```python
from build123d import *

# Parameters (mm, degrees)
SKETCH_W     = 95
SKETCH_H     = 69
SKETCH_R     = 1.5
PAD_DEPTH    = 3
SKETCH001_R  = 4
PAD001_DEPTH = 4
SKETCH002_R  = 1.45
POCKET_DEPTH = 5


with BuildPart() as part:
    # Sketch → Pad (new body)
    with BuildSketch(Plane.XY):
        Rectangle(SKETCH_W, SKETCH_H)
        with Locations((-44, -31)):
            Circle(SKETCH_R, mode=Mode.SUBTRACT)
        with Locations((44, 31)):
            Circle(SKETCH_R, mode=Mode.SUBTRACT)
    extrude(amount=PAD_DEPTH)

    # Sketch001 (on Face8 of Pad) → Pad001 (join)
    with BuildSketch(Plane.XY.offset(3)):
        with Locations((-36.5, 24)):
            Circle(SKETCH001_R)
        with Locations((-36.5, -24)):
            Circle(SKETCH001_R)
        with Locations((36.5, -24)):
            Circle(SKETCH001_R)
        with Locations((36.5, 24)):
            Circle(SKETCH001_R)
    extrude(amount=PAD001_DEPTH)

    # Sketch002 (on Face14 of Pad001) → Pocket (cut)
    with BuildSketch(Plane.XY.offset(7)):
        with Locations((-36.5, 24)):
            Circle(SKETCH002_R)
        with Locations((-36.5, -24)):
            Circle(SKETCH002_R)
        with Locations((36.5, 24)):
            Circle(SKETCH002_R)
        with Locations((36.5, -24)):
            Circle(SKETCH002_R)
    extrude(amount=-POCKET_DEPTH, mode=Mode.SUBTRACT)


solid = part.part
```
For this review, take the finished solid that the model builds, in its own axes (mm). A direction names the side the tool comes from. Give positions to 0.01 mm unless a question says otherwise; leave off trailing zeros. Order: outer loops, then holes, each group sorted by start corner. A loop starts at its lowest first (then second) coordinate and runs counter-clockwise, first axis right, second up.
1) For faces 4 (the face through (-37.65, 23.12, 4.54)), 5 (the face through (38.2, -23.9, 7)), list the 3-axis set-ups (+Z, -Z, +X, -X, +Y, -Y) from which the entire face can be reached by the end or side of a thin tool; tool diameter is ignored.
2) Wall thickness on line 1 (Y direction, x = 36.5, z = 6.05); line 2 (Y direction, x = -44, z = 1.3); line 3 (X direction, y = -25, z = 6.75): over which ranges is each line inside the solid? List them lowest first.
3) Take a section at D-D (y = -24). Give the boundary of the cut face in (x, z), then the cut area to 3 significant figures.
4) Take a section at B-B (x = -44). Give the boundary of the cut face in (y, z), then the cut area to 3 significant figures.
5) The part is to be moulded in two halves that separate along Y. For faces 1 (the face through (-1, -34.5, 1)), 2 (the face through (36, 24, 2)), 3 (the face through (-1, 0, 0)), say which applies: released by +Y, released by -Y, zero draft, split by the parting line, or undercut.
6) Take a section at A-A (z = 5). Give the boundary of the cut face in (x, y), then the cut area to 3 significant figures.
7) Take a section at C-C (y = -31). Give the boundary of the cut face in (x, z), then the cut area to 3 significant figures.
8) Insertion check: pin 1 (1.7 mm diameter, centred on x = 36.5, y = 24, fed in from +Z); pin 2 (2.5 mm diameter, centred on x = -44, y = -31, fed in from -Z); pin 3 (3 mm diameter, centred on x = 6, y = -11.5, fed in from +Z). Each pin has a flat end and moves straight along its axis. Give the tip position at first contact, or say it passes through.
Derived:
1. face 4: +Z
1. face 5: +Z, +X, -X, +Y, -Y
2. line 1: y = -28 to -25.45, -22.55 to -20, 20 to 22.55, 25.45 to 28
2. line 2: y = -34.5 to -32.5, -29.5 to 34.5
2. line 3: x = -40.37 to -37.55, -35.45 to -32.63, 32.63 to 35.45, 37.55 to 40.37
3. outline: (-47.5, 0) - (47.5, 0) - (47.5, 3) - (40.5, 3) - (40.5, 7) - (37.95, 7) - (37.95, 2) - (35.05, 2) - (35.05, 7) - (32.5, 7) - (32.5, 3) - (-32.5, 3) - (-32.5, 7) - (-35.05, 7) - (-35.05, 2) - (-37.95, 2) - (-37.95, 7) - (-40.5, 7) - (-40.5, 3) - (-47.5, 3) - close
3. area: 320 mm2
4. outline: (-34.5, 0) - (-32.5, 0) - (-32.5, 3) - (-34.5, 3) - close; (-29.5, 0) - (34.5, 0) - (34.5, 3) - (-29.5, 3) - close
4. area: 198 mm2
5. face 1: released by -Y
5. face 2: undercut
5. face 3: zero draft
6. outline: circle Ø8 at (-36.5, -24); circle Ø8 at (-36.5, 24); circle Ø8 at (36.5, -24); circle Ø8 at (36.5, 24); hole circle Ø2.9 at (-36.5, -24); hole circle Ø2.9 at (-36.5, 24); hole circle Ø2.9 at (36.5, -24); hole circle Ø2.9 at (36.5, 24)
6. area: 175 mm2
7. outline: (-47.5, 0) - (-45.5, 0) - (-45.5, 3) - (-47.5, 3) - close; (-42.5, 0) - (47.5, 0) - (47.5, 3) - (-42.5, 3) - close
7. area: 276 mm2
8. pin 1: stops at z = 2
8. pin 2: passes through
8. pin 3: stops at z = 3
